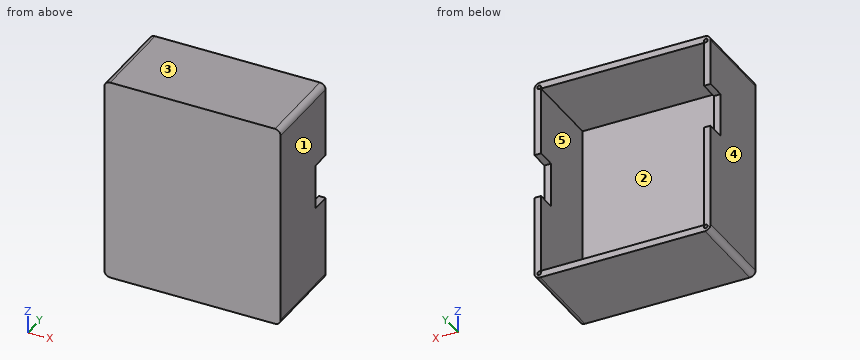
Autodesk Inventor part; units mm, degrees
ref_plane "YZ Plane" through (0, 0, 0) normal (1, 0, 0) x (0, 1, 0)
ref_plane "XZ Plane" through (0, 0, 0) normal (0, 1, 0) x (-1, 0, 0)
ref_plane "XY Plane" through (0, 0, 0) normal (0, 0, 1) x (1, 0, 0)
sketch "Sketch2" plane through (0, 0, 0) normal (0, 1, 0) x (-1, 0, 0)
  line L0 (35.0336, 55.0564) -> (-56.9664, 55.0564)
  line L1 (-56.9664, 55.0564) -> (-56.9664, -51.9436)
  line L2 (-56.9664, -51.9436) -> (35.0336, -51.9436)
  line L3 (35.0336, -51.9436) -> (35.0336, 55.0564)
  point P0 (0, 0)
  dimension "d28" = 107
  dimension "d29" = 92
extrude "Extrusion2" add sketch "Sketch2" along normal blind 45
shell "Shell2" thickness 3.5 removed faces 1 at (-4.367, 45, -16.277)
fillet "Fillet1" radius 3 4 edges at (56.9664, 22.5, 55.0564) (-35.0336, 22.5, 55.0564) (56.9664, 22.5, -51.9436) (-35.0336, 22.5, -51.9436)
sketch "Sketch3" plane through (0, 45, 0) normal (0, 1, 0) x (1, 0, 0)
  circle A0 centre (54.4664, -52.5564) radius 1
  line L0 (-32.0336, -55.0564) -> (53.9664, -55.0564)
  line L1 (56.9664, -52.0564) -> (56.9664, 48.9436)
  line L2 (10.9664, -40.0013) -> (10.9664, -71.8309)
  line L3 (-21.6043, -1.5564) -> (-51.5358, -1.5564)
  circle A1 centre (-32.5336, -52.5564) radius 1
  circle A2 centre (54.4664, 49.4436) radius 1
  circle A3 centre (-32.5336, 49.4436) radius 1
  point P0 (0, 0)
  dimension "d34" = 2
  dimension "d35" = 2.5
  dimension "d36" = 2.5
  dimension "d37" = 46
  dimension "d38" = 53.5
extrude "Extrusion3" cut sketch "Sketch3" against normal blind 7
sketch "Sketch9" plane through (56.9664, 0, 52.0564) normal (1, 0, 0) x (0, 0, -1)
  line L0 (59.45, 45) -> (36.05, 45)
  line L1 (36.05, 45) -> (36.05, 35)
  line L2 (36.05, 35) -> (59.45, 35)
  line L3 (59.45, 35) -> (59.45, 45)
  line L4 (-3, 45) -> (-3, 0)
  line L5 (104, 0) -> (104, 45)
  line L6 (0, 45) -> (101, 45)
  point P0 (52.0564, 0)
  point P1 (-3, 2)
  point P2 (107, 2)
  dimension "d102" = 10
  dimension "d103" = 39.05
  dimension "d104" = 44.55
  dimension "d105" = 0
extrude "Extrusion5" cut sketch "Sketch9" against normal blind 8
sketch "Sketch10" plane through (-35.0336, 0, -48.9436) normal (-1, 0, 0) x (0, 0, 1)
  line L0 (54.05, 35) -> (76.95, 35)
  line L1 (76.95, 35) -> (76.95, 45)
  line L2 (76.95, 45) -> (54.05, 45)
  line L3 (54.05, 45) -> (54.05, 35)
  line L4 (104, 0) -> (104, 45)
  line L5 (0, 45) -> (101, 45)
  line L6 (-3, 45) -> (-3, 0)
  point P0 (48.9436, 0)
  point P1 (107, 2)
  point P2 (-3, 2)
  dimension "d108" = 27.05
  dimension "d109" = 0
  dimension "d110" = 57.05
  dimension "d111" = 10
extrude "Extrusion6" cut sketch "Sketch10" against normal blind 8
properties part number "MotorDriverModel"
Geometry: final body of the model. Coordinates: model frame, mm. Face numbers are marked on the shaded views. A direction names the side the tool comes from. Give positions to 0.01 mm unless a question says otherwise; leave off trailing zeros. Loops run counter-clockwise (first coordinate to the right, second up) from the corner with the lowest first, then second, coordinate; pieces in that order, holes last. Notation, with made-up numbers: (40, 69) -> (66, 69) arc R24 cw to (66, 97) -> close; hole circle Ø4 at (48.5, 65). An arc over 180 degrees is marked (long way). Use one line per item in the form item = value.
Item 1: Section query C-C on y = 40. Output: boundary loops of the cut face in (x, z), and give its area (3 significant figures).
A:
outline = (-35.03, -48.94) arc R3 ccw to (-32.03, -51.94) -> (53.97, -51.94) arc R3 ccw to (56.97, -48.94) -> (56.97, -7.39) -> (53.47, -7.39) -> (53.47, -48.44) -> (-31.53, -48.44) -> (-31.53, 5.11) -> (-35.03, 5.11) -> close; (-35.03, 28.01) -> (-31.53, 28.01) -> (-31.53, 51.56) -> (53.47, 51.56) -> (53.47, 16.01) -> (56.97, 16.01) -> (56.97, 52.06) arc R3 ccw to (53.97, 55.06) -> (-32.03, 55.06) arc R3 ccw to (-35.03, 52.06) -> close; hole circle Ø2 at (-32.53, -49.44); hole circle Ø2 at (-32.53, 52.56); hole circle Ø2 at (54.47, -49.44); hole circle Ø2 at (54.47, 52.56)
area = 1,160 mm^2
Item 2: Line query: probe 1 along Z at (x, y) = (25, 13); probe 2 along X at (y, z) = (24, -5.5); probe 3 along Y at (x, z) = (-10, -15). Output: solid intervals per line, ascending.
A:
probe_1 = -51.94 to -48.44, 51.56 to 55.06
probe_2 = -35.03 to -31.53, 53.47 to 56.97
probe_3 = 0 to 3.5
Item 3: Access query for the marked faces 4 and 5. Directions: +Z, -Z, +X, -X, +Y, -Y. A direction counts if a zero-diameter tool reaches every point of the face in a straight line with its end or side. Return the directions, or none.
A:
face_4 = +Z, -Z, -X, +Y, -Y
face_5 = +Y
Item 4: Section query A-A on z = -14. Output: boundary loops of the cut face in (x, y), and give its area (4 significant figures).
A:
outline = (-35.03, 0) -> (56.97, 0) -> (56.97, 45) -> (53.47, 45) -> (53.47, 3.5) -> (-31.53, 3.5) -> (-31.53, 45) -> (-35.03, 45) -> close
area = 612.5 mm^2
Item 5: Draft query along X for the marked faces 1, 2 and 3. Return one class per face: pulls with the +X half, pulls with the -X half, needs draft (parallel to the pull), parting line crosses it, or undercut.
A:
face_1 = pulls with the +X half
face_2 = undercut
face_3 = needs draft
Item 6: Section query B-B on x = -17. Output: boundary loops of the cut face in (y, z).
A:
outline = (0, -51.94) -> (45, -51.94) -> (45, -48.44) -> (3.5, -48.44) -> (3.5, 51.56) -> (45, 51.56) -> (45, 55.06) -> (0, 55.06) -> close
Item 7: Section query D-D on y = 25. Output: boundary loops of the cut face in (x, z), and give its area (3 significant figures).
A:
outline = (-35.03, -48.94) arc R3 ccw to (-32.03, -51.94) -> (53.97, -51.94) arc R3 ccw to (56.97, -48.94) -> (56.97, 52.06) arc R3 ccw to (53.97, 55.06) -> (-32.03, 55.06) arc R3 ccw to (-35.03, 52.06) -> close; hole (-31.53, -48.44) -> (53.47, -48.44) -> (53.47, 51.56) -> (-31.53, 51.56) -> close
area = 1,340 mm^2
Item 8: Pin query (flat end, axial travel): P1, Ø3, axis at x = 24, z = 13, coming from the +Y side; P2, Ø4, axis at x = -33, z = 20.5, coming from the +Y side; P3, Ø0.6, axis at x = -32, z = -49.5, coming from the +Y side. Return the tip coordinate at first contact, or that it passes through.
A:
P1 = 3.5
P2 = 35
P3 = 38
